from build123d import *

# Parameters (mm, degrees)
SKETCH_R           = 13.063078
PAD_DEPTH          = 4
SKETCH001_R        = 0.961125
POCKET_DEPTH       = 78.328708
POLARPATTERN_COUNT = 5
SKETCH002_R        = 5.538718
PAD001_DEPTH       = 6
SKETCH003_R        = 3.898849
POCKET001_DEPTH    = 10.001


with BuildPart() as part:
    # Sketch → Pad (new body)
    with BuildSketch(Plane.XY):
        Circle(SKETCH_R)
    extrude(amount=PAD_DEPTH)

    # Sketch001 (on DatumPlane) → Pocket (cut, through all)
    with BuildSketch(Plane.XY.offset(4)):
        with Locations((0, 9.326428)):
            Circle(SKETCH001_R)
    pocket = extrude(amount=-POCKET_DEPTH, mode=Mode.SUBTRACT)

    # PolarPattern: Pocket ×5 about axis
    polarpattern_axis = Axis((0, 0, 4), (0, 0, 1))
    for i in range(1, POLARPATTERN_COUNT):
        add(pocket.rotate(polarpattern_axis, i * 360 / POLARPATTERN_COUNT), mode=Mode.SUBTRACT)

    # Sketch002 (on DatumPlane) → Pad001 (join)
    with BuildSketch(Plane.XY.offset(4)):
        Circle(SKETCH002_R)
    extrude(amount=PAD001_DEPTH)

    # Sketch003 (on DatumPlane) → Pocket001 (cut, through all)
    with BuildSketch(Plane.XY.offset(10)):
        Circle(SKETCH003_R)
    extrude(amount=-POCKET001_DEPTH, mode=Mode.SUBTRACT)


solid = part.part
CAD build for the part. Positions are in the model's coordinates, mm. A direction names the side the tool comes from. Coordinates: 2 decimals unless noted, no trailing zeros. Order: outer loops, then holes, each group sorted by start corner. A loop starts at its lowest first (then second) coordinate and runs counter-clockwise, first axis right, second up.
Item 1: Band-saw the part on C-C on y = 2.75. List the corners of the cut face in (x, z).
Check sheet entries:
outline: (-12.77, 0) - (-9.82, 0) - (-9.82, 4) - (-12.77, 4) - close; (-7.92, 0) - (-2.76, 0) - (-2.76, 10) - (-4.81, 10) - (-4.81, 4) - (-7.92, 4) - close; (2.76, 0) - (7.92, 0) - (7.92, 4) - (4.81, 4) - (4.81, 10) - (2.76, 10) - close; (9.82, 0) - (12.77, 0) - (12.77, 4) - (9.82, 4) - close
Item 2: 3-axis set-ups, long thin cutter, end or side, ignore diameter. For faces 1 (the face through (8.196, 2.197, 2.028)), 2 (the face through (-4.395, -3.37, 6.958)): which of +Z, -Z, +X, -X, +Y, -Y reach the whole face in a straight line?
Check sheet entries:
face 1: +Z, -Z
face 2: +Z
Item 3: Band-saw the part on A-A on x = 0. List the corners of the cut face in (y, z), plus the area to 3 significant figures.
Check sheet entries:
outline: (-13.06, 0) - (-3.9, 0) - (-3.9, 10) - (-5.54, 10) - (-5.54, 4) - (-13.06, 4) - close; (3.9, 0) - (8.37, 0) - (8.37, 4) - (5.54, 4) - (5.54, 10) - (3.9, 10) - close; (10.29, 0) - (13.06, 0) - (13.06, 4) - (10.29, 4) - close
area: 85.3 mm2
Item 4: Pin check, flat tips, straight feed: pin 1 Ø5 at (x, y) = (8, -3) entering from -Z; pin 2 Ø5 at (y, z) = (3, 8) entering from -X; pin 3 Ø2 at (x, y) = (8.87, 2.88) entering from +Z; pin 4 Ø6 at (y, z) = (-5.5, 3.5) entering from +X. Stop position of each tip, or through.
Check sheet entries:
pin 1: stops at z = 0
pin 2: stops at x = -5.52
pin 3: stops at z = 4
pin 4: stops at x = 12.82
Item 5: Two-plate mould, pull along Y, no slides. Class faces 3 (the face through (0, -6, 4)), 4 (the face through (-2.832, -12.752, 1.972)), 5 (the face through (-9.815, 3.058, 2.028)): +Y half, -Y half, draft (parallel to the pull), parting line (faces both ways), or undercut.
Check sheet entries:
face 3: draft
face 4: parting line
face 5: undercut
Item 6: Band-saw the part on B-B on y = 0. List the corners of the cut face in (x, z), plus the area to 3 significant figures.
Check sheet entries:
outline: (-13.06, 0) - (-3.9, 0) - (-3.9, 10) - (-5.54, 10) - (-5.54, 4) - (-13.06, 4) - close; (3.9, 0) - (13.06, 0) - (13.06, 4) - (5.54, 4) - (5.54, 10) - (3.9, 10) - close
area: 93.0 mm2
Item 7: Band-saw the part on D-D on z = 7.25. List the corners of the cut face in (x, y).
Check sheet entries:
outline: circle Ø11.08 at (0, 0); hole circle Ø7.8 at (0, 0)
Item 8: Drill centre lines: L1, parallel to Y at x = 0, z = 2.4; L2, parallel to Z at x = -4.25, y = 4.75; L3, parallel to Y at x = -3.25, z = 2.75. Where is each one in solid material? Low to high.
Check sheet entries:
L1: y = -13.06 to -3.9, 3.9 to 8.37, 10.29 to 13.06
L2: z = 0 to 4
L3: y = -12.65 to -2.15, 2.15 to 12.65
